```python
from build123d import *

# Parameters (mm, degrees)
SKETCH_1_W          = 40
SKETCH_1_H          = 435
SKETCH_1_H_2        = 40
SKETCH_1_W_2        = 120
EXTRUDE_1_DEPTH     = 5
CUT_EXTRUDE_2_DEPTH = 498.041245773
SKETCH_3_W          = 5
SKETCH_3_H          = 20
CUT_EXTRUDE_3_DEPTH = 466.886252212
SKETCH_4_R          = 1
CUT_EXTRUDE_4_DEPTH = 305.836021494


with BuildPart() as part:
    # 草图1 → 凸台-拉伸1 (new body)
    with BuildSketch(Plane(origin=(0, 0, 0), x_dir=(1, 0, 0), z_dir=(0, 1, 0))):
        with Locations((-80, 237.5)):
            Rectangle(SKETCH_1_W, SKETCH_1_H)
        with Locations((-80, 0)):
            Rectangle(SKETCH_1_W, SKETCH_1_H_2)
        Rectangle(SKETCH_1_W_2, SKETCH_1_H_2)
        with Locations((80, 0)):
            Rectangle(SKETCH_1_W, SKETCH_1_H_2)
        with Locations((80, 237.5)):
            Rectangle(SKETCH_1_W, SKETCH_1_H)
    extrude(amount=EXTRUDE_1_DEPTH)

    # 草图2 → 切除-拉伸2 (cut, through all)
    with BuildSketch(Plane(origin=(100, 0, 0), x_dir=(0, 0, -1), z_dir=(1, 0, 0))):
        Polygon((155, 5), (455, 1), (455, 5), align=None)
    extrude(amount=-CUT_EXTRUDE_2_DEPTH, mode=Mode.SUBTRACT)

    # 草图3 → 切除-拉伸3 (cut, through all)
    with BuildSketch(Plane(origin=(0, 5, 0), x_dir=(1, 0, 0), z_dir=(0, 1, 0))):
        Polygon((-100, 455), (-100, 230), (-95, 230), (-90, 230), (-85, 230), (-80, 230), (-75, 230), (-70, 230), (-65, 230), (-60, 230), (60, 230), (65, 230), (70, 230), (75, 230), (80, 230), (85, 230), (90, 230), (95, 230), (100, 230), (100, 455), align=None)
        with Locations((-92.5, 220)):
            Rectangle(SKETCH_3_W, SKETCH_3_H)
        with Locations((-82.5, 220)):
            Rectangle(SKETCH_3_W, SKETCH_3_H)
        with Locations((-72.5, 220)):
            Rectangle(SKETCH_3_W, SKETCH_3_H)
        with Locations((-62.5, 220)):
            Rectangle(SKETCH_3_W, SKETCH_3_H)
        with Locations((62.5, 220)):
            Rectangle(SKETCH_3_W, SKETCH_3_H)
        with Locations((72.5, 220)):
            Rectangle(SKETCH_3_W, SKETCH_3_H)
        with Locations((82.5, 220)):
            Rectangle(SKETCH_3_W, SKETCH_3_H)
        with Locations((92.5, 220)):
            Rectangle(SKETCH_3_W, SKETCH_3_H)
    extrude(amount=-CUT_EXTRUDE_3_DEPTH, mode=Mode.SUBTRACT)

    # 草图4 → 切除-拉伸4 (cut, through all)
    with BuildSketch(Plane(origin=(100, 0, 0), x_dir=(0, 0, -1), z_dir=(1, 0, 0))):
        with Locations((225, 2)):
            Circle(SKETCH_4_R)
        with Locations((220, 2)):
            Circle(SKETCH_4_R)
        with Locations((215, 2)):
            Circle(SKETCH_4_R)
    extrude(amount=-CUT_EXTRUDE_4_DEPTH, mode=Mode.SUBTRACT)


solid = part.part
```
Design review of the part built by this model. Coordinates are the model's own, in mm. A direction names the side the tool comes from. Give positions to 0.01 mm unless a question says otherwise; leave off trailing zeros. Order: outer loops, then holes, each group sorted by start corner. A loop starts at its lowest first (then second) coordinate and runs counter-clockwise, first axis right, second up. Notation, with made-up numbers: (9.25, -35.75) -> (35.25, -35.75) arc R26 cw to (35.25, -2.75) -> close; hole circle Ø3 at (-5, -8). An arc over 180 degrees is marked (long way). Write item = value, one per line. Start each with the question number.
(1) Mouldability with a two-part tool opening along X and no side actions: class faces 1 (the face through (-100, 2, -107)), 2 (the face through (100, 2, -103)), 3 (the face through (60, 2, -114)), 4 (the face through (-1, 5, -10)) as +X half, -X half, draft (parallel to the pull), parting line (faces both ways), or undercut.
(2) For pin 1 (2 mm diameter, centred on x = -82.5, y = 1.5, fed in from -Z); pin 2 (1.5 mm diameter, centred on x = 9.5, y = 1.5, fed in from -Z), all flat-tipped, find the tip position at first contact; note any pin that passes through.
(3) We need section A-A on z = -146.5. Write out the cut boundary in (x, y).
(4) To check wall thickness, follow line 1 along X through (y, z) = (2.05, -68.5); line 2 along Z through (x, y) = (-69.5, 2.55); line 3 along Z through (x, y) = (-11, 2.1). State the ranges of each line that lie inside material, in increasing order.
(5) We need section B-B on y = 2. State how many separate pieces and enclosed holes the cut face has, plus the area to 3 significant figures.
(6) We need section C-C on x = 56. Write out the cut boundary in (y, z).
(7) For faces 5 (the face through (1, 2, -20)), 6 (the face through (65, 0, -79)), list the 3-axis set-ups (+Z, -Z, +X, -X, +Y, -Y) from which the entire face can be reached by the end or side of a thin tool; tool diameter is ignored.
Numbers:
q1.face_1 = -X half
q1.face_2 = +X half
q1.face_3 = undercut
q1.face_4 = draft
q2.pin_1 = -210
q2.pin_2 = -20
q3.outline = (-100, 0) -> (-60, 0) -> (-60, 5) -> (-100, 5) -> close; (60, 0) -> (100, 0) -> (100, 5) -> (60, 5) -> close
q4.line_1 = -100 to -60, 60 to 100
q4.line_2 = -230 to -225.84, -224.16 to -220.84, -219.16 to -215.84, -214.16 to 20
q4.line_3 = -20 to 20
q5.separate_pieces = 25
q5.enclosed_holes = 0
q5.area = 23,800 mm^2
q6.outline = (0, -20) -> (5, -20) -> (5, 20) -> (0, 20) -> close
q7.face_5 = -Z, +Y, -Y
q7.face_6 = +Z, -Z, +X, -X, -Y
